```python
from build123d import *

# Parameters (mm, degrees)
ESQUISSE5_W                  = 14
ESQUISSE5_H                  = 44
BOSS_EXTRU_2_DEPTH           = 5
BOSS_EXTRU_3_DEPTH           = 60
ENL_V_MAT_EXTRU_2_DEPTH      = 80.730797061
ENL_V_MAT_EXTRU_2_DEPTH_BACK = 80.730797061
ESQUISSE8_R                  = 1.6
ESQUISSE10_R                 = 2.05
ESQUISSE10_W                 = 20
ESQUISSE10_H                 = 40
ESQUISSE10_R_2               = 1.6
ENL_V_MAT_EXTRU_3_DEPTH      = 80.730797061
ESQUISSE11_R                 = 2.05
ENL_V_MAT_EXTRU_4_DEPTH      = 76.709972923
CONG_3_R                     = 1.5


with BuildPart() as part:
    # Esquisse5 → Boss.-Extru.2 (new body)
    with BuildSketch(Plane(origin=(0, 0, 0), x_dir=(1, 0, 0), z_dir=(0, 1, 0))):
        with Locations((7, 22)):
            Rectangle(ESQUISSE5_W, ESQUISSE5_H)
    extrude(amount=BOSS_EXTRU_2_DEPTH)

    # Esquisse6 → Boss.-Extru.3 (add)
    with BuildSketch(Plane(origin=(0, 5, 0), x_dir=(1, 0, 0), z_dir=(0, 1, 0))):
        Polygon((9, 15), (9, 0), (14, 0), (14, 20), (5, 20), (5, 44), (0, 44), (0, 15), align=None)
    extrude(amount=BOSS_EXTRU_3_DEPTH)

    # Esquisse8 → Enlèv. mat.-Extru.2 (cut, two sides: drawn at the far end of the back side and taken through both)
    with BuildSketch(Plane(origin=(0, 0, 0), x_dir=(0, 0, -1), z_dir=(1, 0, 0)).offset(-ENL_V_MAT_EXTRU_2_DEPTH_BACK)):
        with Locations((30, 25)):
            Circle(ESQUISSE8_R)
        with Locations((10, 45)):
            Circle(ESQUISSE8_R)
    extrude(amount=ENL_V_MAT_EXTRU_2_DEPTH + ENL_V_MAT_EXTRU_2_DEPTH_BACK, mode=Mode.SUBTRACT)

    # Esquisse10 → Enlèv. mat.-Extru.3 (cut, through all)
    # profile 1 of 5: a face of its own
    with BuildSketch(Plane.ZY):
        with Locations((-25, 11)):
            Circle(ESQUISSE10_R)
    # profile 2 of 5: a face of its own
    with BuildSketch(Plane.ZY):
        with Locations((-35, 11)):
            Circle(ESQUISSE10_R)
    # profile 3 of 5: a face of its own
    with BuildSketch(Plane.ZY):
        with Locations((-30, 35)):
            Rectangle(ESQUISSE10_W, ESQUISSE10_H)
        with Locations((-30, 25)):
            Circle(ESQUISSE10_R_2, mode=Mode.SUBTRACT)
    # profile 4 of 5: a face of its own
    with BuildSketch(Plane.ZY):
        with Locations((-25, 59)):
            Circle(ESQUISSE10_R)
    # profile 5 of 5: a face of its own
    with BuildSketch(Plane.ZY):
        with Locations((-35, 59)):
            Circle(ESQUISSE10_R)
    extrude(amount=-ENL_V_MAT_EXTRU_3_DEPTH, mode=Mode.SUBTRACT)

    # Esquisse11 → Enlèv. mat.-Extru.4 (cut, through all)
    with BuildSketch(Plane(origin=(0, 5, 0), x_dir=(1, 0, 0), z_dir=(0, 1, 0))):
        with Locations(Location((9.5, 39.5, 0), (0, 0, 270))):
            Circle(ESQUISSE11_R)
        with Locations(Location((4.5, 4.5, 0), (0, 0, 270))):
            Circle(ESQUISSE11_R)
    extrude(amount=-ENL_V_MAT_EXTRU_4_DEPTH, mode=Mode.SUBTRACT)

    # Congé3
    cong_3_edges = [part.edges().sort_by_distance(p)[0] for p in [
        (0, 5, -7.5),
        (4.5, 65, -15),
        (0, 35, -15),
        (9, 65, -7.5),
        (9, 35, -15),
        (9, 35, 0),
        (2.5, 65, -44),
        (0, 65, -29.5),
        (11.5, 65, 0),
        (9.5, 5, -20),
        (9, 5, -7.5),
        (4.5, 5, -15),
        (4.5, 5, 0),
        (0, 2.5, 0),
        (0, 32.5, -44),
    ]]
    fillet(cong_3_edges, radius=CONG_3_R)


solid = part.part
```
Design review of the part built by this model. Coordinates are the model's own, in mm. A direction names the side the tool comes from. Give positions to 0.01 mm unless a question says otherwise; leave off trailing zeros. Order: outer loops, then holes, each group sorted by start corner. A loop starts at its lowest first (then second) coordinate and runs counter-clockwise, first axis right, second up. Notation, with made-up numbers: (62.5, -25.75) -> (76.5, -25.75) arc R27 ccw to (76.5, -0.75) -> close; hole circle Ø9 at (11.25, 14.5). An arc over 180 degrees is marked (long way). Write item = value, one per line. Start each with the question number.
(1) For pin 1 (3.5 mm diameter, centred on y = 47, z = -5.5, fed in from -X); pin 2 (1.5 mm diameter, centred on x = 7.5, y = 23, fed in from +Z); pin 3 (5 mm diameter, centred on x = 6.5, y = 7, fed in from +Z), all flat-tipped, find the tip position at first contact; note any pin that passes through.
(2) We need section C-C on y = 26. Write out the cut boundary in (x, z), plus the area to 3 significant figures.
(3) For faces 1 (the face through (0.45, 35.4, -15.43)), 2 (the face through (8.253, 2.535, -41.127)), 3 (the face through (2, 15, -30)), list the 3-axis set-ups (+Z, -Z, +X, -X, +Y, -Y) from which the entire face can be reached by the end or side of a thin tool; tool diameter is ignored.
(4) We need section D-D on z = -25. Write out the cut boundary in (x, y), plus the area to 3 significant figures.
(5) We need section B-B on y = 11. Write out the cut boundary in (x, z), plus the area to 3 significant figures.
(6) We need section A-A on z = -10. Write out the cut boundary in (x, y).
(7) Mouldability with a two-part tool opening along Z and no side actions: class faces 4 (the face through (3.23, 64.57, -43.55)), 5 (the face through (3.253, 2.535, -6.127)), 6 (the face through (2.465, 61.033, -25.267)), 7 (the face through (11, 27, 0)) as +Z half, -Z half, draft (parallel to the pull), parting line (faces both ways), or undercut.
(8) To check wall thickness, follow line 1 along Y through (x, z) = (1.45, -35); line 2 along Z through (x, y) = (2.5, 46); line 3 along X through (y, z) = (1.2, -39.5). State the ranges of each line that lie inside material, in increasing order.
Numbers:
q1.pin_1 = 9
q1.pin_2 = -14.8
q1.pin_3 = -0.38
q2.outline = (0, -42.5) arc R1.5 ccw to (1.5, -44) -> (5, -44) -> (5, -40) -> (0, -40) -> close; (0, -20) -> (14, -20) -> (14, 0) -> (10.5, 0) arc R1.5 ccw to (9, -1.5) -> (9, -13.5) arc R1.5 cw to (7.5, -15) -> (1.5, -15) arc R1.5 ccw to (0, -16.5) -> close
q2.area = 164 mm^2
q3.face_1 = +Z, -X, +Y
q3.face_2 = +Y, -Y
q3.face_3 = +X, -X
q4.outline = (0, 0) -> (14, 0) -> (14, 5) -> (5, 5) -> (5, 8.95) -> (0, 8.95) -> close; (0, 13.05) -> (5, 13.05) -> (5, 15) -> (0, 15) -> close; (0, 55) -> (5, 55) -> (5, 56.95) -> (0, 56.95) -> close; (0, 61.05) -> (5, 61.05) -> (5, 65) -> (1.5, 65) arc R1.5 ccw to (0, 63.5) -> close
q4.area = 129 mm^2
q5.outline = (0, -42.5) arc R1.5 ccw to (1.5, -44) -> (5, -44) -> (5, -37.05) -> (0, -37.05) -> close; (0, -32.95) -> (5, -32.95) -> (5, -27.05) -> (0, -27.05) -> close; (0, -22.95) -> (5, -22.95) -> (5, -20) -> (14, -20) -> (14, 0) -> (10.5, 0) arc R1.5 ccw to (9, -1.5) -> (9, -13.5) arc R1.5 cw to (7.5, -15) -> (1.5, -15) arc R1.5 ccw to (0, -16.5) -> close
q5.area = 223 mm^2
q6.outline = (0, 0) -> (14, 0) -> (14, 43.4) -> (9, 43.4) -> (9, 6.5) arc R1.5 cw to (7.5, 5) -> (1.5, 5) arc R1.5 ccw to (0, 3.5) -> close; (9, 46.6) -> (14, 46.6) -> (14, 65) -> (10.5, 65) arc R1.5 ccw to (9, 63.5) -> close
q7.face_4 = -Z half
q7.face_5 = undercut
q7.face_6 = undercut
q7.face_7 = +Z half
q8.line_1 = 0 to 8.95, 13.05 to 15, 55 to 56.95, 61.05 to 65
q8.line_2 = -44 to -40, -20 to -15
q8.line_3 = 0 to 7.45, 11.55 to 14
